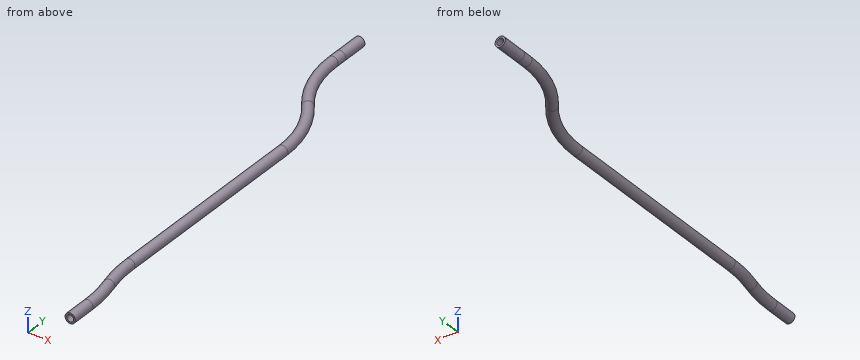
```python
from build123d import *
from build123d.topology import SkipClean

# Parameters (mm, degrees)
SKETCH_1_R      = 3
SKETCH_1_R_2    = 2
EXTRUDE_1_DEPTH = 15
SKETCH_1_2_R    = 3
SKETCH_1_2_R_2  = 2


with BuildPart() as part:
    # Sketch 1 → Extrude 1 (new body)
    with BuildSketch(Plane(origin=(0, 0, 0), x_dir=(1, 0, 0), z_dir=(0, 1, 0))):
        with Locations(Location((0, 0, 0), (0, 0, 270))):
            Circle(SKETCH_1_R)
        with Locations(Location((0, 0, 0), (0, 0, 270))):
            Circle(SKETCH_1_R_2, mode=Mode.SUBTRACT)
    extrude(amount=EXTRUDE_1_DEPTH)

    # Sweep 1: sweep along a path in Sketch 296
    with SkipClean():  # the faces are left unmerged after this step: merging them gives an invalid solid
        with BuildLine(Plane.XY) as sweep_1_path:
            Line((0, 0), (0, -6))
            ThreePointArc((0, -6), (3.369619461, -25.824227602), (13.1, -43.421785099))
            ThreePointArc((13.1, -43.421785099), (22.830380539, -61.019342597), (26.2, -80.843570198))
            Line((26.2, -80.843570198), (26.2, -201.157300532))
            ThreePointArc((26.2, -201.157300532), (26.827460668, -211.157300532), (28.7, -221.000435365))
            ThreePointArc((28.7, -221.000435365), (30.572539332, -230.843570198), (31.2, -240.843570198))
            Line((31.2, -240.843570198), (31.2, -254.843570198))
        # Sketch 1_2 → Sweep 1 (sweep)
        with BuildSketch(Plane(origin=(0, 0, 0), x_dir=(1, 0, 0), z_dir=(0, 1, 0))):
            Circle(SKETCH_1_2_R)
            Circle(SKETCH_1_2_R_2, mode=Mode.SUBTRACT)
        sweep(path=sweep_1_path.line)


solid = part.part
```
Can you work these out from the model? Positions are in its coordinate system, mm. Give positions to 0.01 mm unless a question says otherwise; leave off trailing zeros. Loops run counter-clockwise (first coordinate to the right, second up) from the corner with the lowest first, then second, coordinate; pieces in that order, holes last. Notation, with made-up numbers: M 57.25,71 L 95.25,71 A33 cw 95.25,101 Z; hole C 2,77.5 d2. An arc over 180 degrees is marked long. Use CSV: the item, a comma, the result in double quotes. Start each with the question number.
1. For P1, Ø3, axis at y = -161.5, z = 1.5, coming from the -X side, with a flat end and sliding along its axis, tell me the tip position at first contact or that it passes through.
2. Imagine slicing it at B-B, the plane y = -134.5. Write out the boundary of the cut face in (x, z).
3. If I drill on L1, parallel to X at y = -154.5, z = 0; L2, parallel to Z at x = 0, y = 7, over which ranges is the centre line in solid material (lowest first)?
Response values:
1,P1,"x = 23.2"
2,outline,"C 26.2,0 d6; hole C 26.2,0 d4"
3,L1,"23.2 to 24.2, 28.2 to 29.2"
3,L2,"-3 to -2, 2 to 3"
